Input: dimensioned drawing with shaded views. Units: mm. Origin: part minimum x, y, z. Coordinates: 2 decimals unless noted, no trailing zeros. Loops run counter-clockwise (first coordinate to the right, second up) from the corner with the lowest first, then second, coordinate; pieces in that order, holes last.
Item 1: Contact query for a flat-ended pin moving along its axis: P1, Ø21.5, axis at x = 31.75, y = 76.2, coming from the -Z side. Output: stop coordinate, or through.
Item 2: Section B-B on y = 76.2. Return loops of the section in (x, z).
Item 3: Section C-C on x = 31.75. Return loops of the section in (y, z).
Item 4: Section D-D on z = 1.7. Return loops of the section in (x, y), and give its area (3 significant figures).
Item 5: Ray query, line 1 along Y through (x, z) = (12.7, 1.65) (1 decimal); line 2 along Y through (x, z) = (31.75, 1.7); line 3 along X through (y, z) = (13, 3.2). Return the intervals inside material, ascending.
Item 6: Section A-A on y = 10.16. Return loops of the section in (x, z), and give its area (3 significant figures).
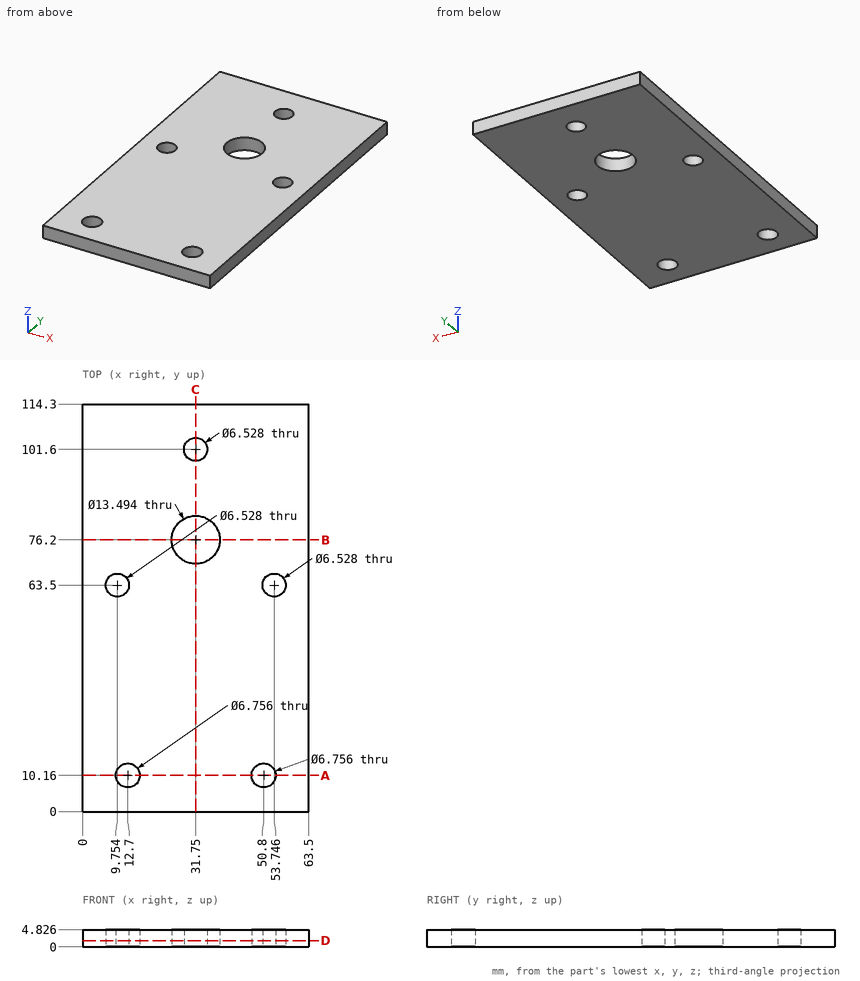
Results found:
1. P1: stops at z = 0
2. outline: (0, 0) - (25, 0) - (25, 4.83) - (0, 4.83) - close; (38.5, 0) - (63.5, 0) - (63.5, 4.83) - (38.5, 4.83) - close
3. outline: (0, 0) - (69.45, 0) - (69.45, 4.83) - (0, 4.83) - close; (82.95, 0) - (98.34, 0) - (98.34, 4.83) - (82.95, 4.83) - close; (104.86, 0) - (114.3, 0) - (114.3, 4.83) - (104.86, 4.83) - close
4. outline: (0, 0) - (63.5, 0) - (63.5, 114.3) - (0, 114.3) - close; hole circle Ø6.53 at (9.75, 63.5); hole circle Ø6.76 at (12.7, 10.16); hole circle Ø13.49 at (31.75, 76.2); hole circle Ø6.53 at (31.75, 101.6); hole circle Ø6.76 at (50.8, 10.16); hole circle Ø6.53 at (53.75, 63.5)
4. area: 6,940 mm2
5. line 1: y = 0 to 6.8, 13.5 to 62.1, 64.9 to 114.3
5. line 2: y = 0 to 69.45, 82.95 to 98.34, 104.86 to 114.3
5. line 3: x = 0 to 10.87, 14.53 to 48.97, 52.63 to 63.5
6. outline: (0, 0) - (9.32, 0) - (9.32, 4.83) - (0, 4.83) - close; (16.08, 0) - (47.42, 0) - (47.42, 4.83) - (16.08, 4.83) - close; (54.18, 0) - (63.5, 0) - (63.5, 4.83) - (54.18, 4.83) - close
6. area: 241 mm2
